```python
from build123d import *

# Parameters (mm, degrees)
SKETCH1_W           = 220
SKETCH1_H           = 220
BOSS_EXTRUDE1_DEPTH = 200
FILLET1_R           = 10
SKETCH2_R           = 30
CUT_EXTRUDE1_DEPTH  = 20
SKETCH3_W           = 80
SKETCH3_H           = 36
CUT_EXTRUDE2_DEPTH  = 20
SKETCH4_W           = 13.191247326
SKETCH4_H           = 23.565374265
CUT_EXTRUDE3_DEPTH  = 10


with BuildPart() as part:
    # Sketch1 → Boss-Extrude1 (new body)
    with BuildSketch(Plane(origin=(0, 0, 0), x_dir=(1, 0, 0), z_dir=(0, 1, 0))):
        Rectangle(SKETCH1_W, SKETCH1_H)
    extrude(amount=BOSS_EXTRUDE1_DEPTH)

    # Fillet1
    fillet1_edges = [part.edges().sort_by_distance(p)[0] for p in [
        (110, 100, 110),
        (-110, 100, 110),
        (-110, 100, -110),
        (110, 100, -110),
    ]]
    fillet(fillet1_edges, radius=FILLET1_R)

    # Sketch2 → Cut-Extrude1 (cut)
    with BuildSketch(Plane.XZ):
        with Locations((0, -50)):
            Circle(SKETCH2_R)
        with Locations((0, 60)):
            Circle(SKETCH2_R)
    extrude(amount=-CUT_EXTRUDE1_DEPTH, mode=Mode.SUBTRACT)

    # Sketch3 → Cut-Extrude2 (cut)
    with BuildSketch(Plane.XY.offset(110)):
        with Locations((0, 162)):
            Rectangle(SKETCH3_W, SKETCH3_H)
    extrude(amount=-CUT_EXTRUDE2_DEPTH, mode=Mode.SUBTRACT)

    # Sketch4 → Cut-Extrude3 (cut)
    with BuildSketch(Plane.ZY.offset(-40)):
        with Locations((100, 164.204493947)):
            Rectangle(SKETCH4_W, SKETCH4_H)
    extrude(amount=-CUT_EXTRUDE3_DEPTH, mode=Mode.SUBTRACT)


solid = part.part
```
Read the model definition and answer for the solid it produces. Units are mm, in the model's axes. A direction names the side the tool comes from. Coordinates: 2 decimals unless noted, no trailing zeros. Write each loop counter-clockwise with the first axis right and the second up, starting at its lowest first coordinate (ties: lowest second). Pieces come first, ordered by that corner, then holes. Notation, with made-up numbers: (88, -3) -> (96, -3) arc R19 ccw to (96, 24) -> close; hole circle Ø8 at (77, -31). An arc over 180 degrees is marked (long way). Answer as a JSON object with one key per item and string values.
Q1. Determine the mould class of faces 1 (the flat face through (-1, 99, -110)), 2 (the flat face through (45, 175.987, 100)), 3 (the flat face through (-40, 162, 100)) for opening direction Z: pulls with the +Z half, pulls with the -Z half, needs draft (parallel to the pull), parting line crosses it, or undercut.
The answers:
{"face 1": "pulls with the -Z half", "face 2": "undercut", "face 3": "needs draft"}
Q2. The part is cut by section A-A on y = 13. Give the vertices of the cut face in (x, z).
The answers:
{"outline": "(-110, -100) arc R10 ccw to (-100, -110) -> (100, -110) arc R10 ccw to (110, -100) -> (110, 100) arc R10 ccw to (100, 110) -> (-100, 110) arc R10 ccw to (-110, 100) -> close; hole circle Ø60 at (0, -50); hole circle Ø60 at (0, 60)"}
Q3. The part is cut by section C-C on x = 0. Give the vertices of the cut face in (y, z).
The answers:
{"outline": "(0, -110) -> (200, -110) -> (200, 110) -> (180, 110) -> (180, 90) -> (144, 90) -> (144, 110) -> (0, 110) -> (0, 90) -> (20, 90) -> (20, 30) -> (0, 30) -> (0, -20) -> (20, -20) -> (20, -80) -> (0, -80) -> close"}
Q4. Consider line 1 (Z direction, x = 0, y = 12.5); line 2 (X direction, y = 18.5, z = 45.5); line 3 (X direction, y = 13, z = 100.5). Determine where each line is inside the solid, lowest interval first. Write a range as [from, to].
The answers:
{"line 1": "z = [-110, -80], [-20, 30], [90, 110]", "line 2": "x = [-110, -26.26], [26.26, 110]", "line 3": "x = [-109.99, 109.99]"}
Q5. A tool of negligible diameter and unlimited length cuts with its end or side. For faces 4 (the flat face through (45, 164, 106.596)), 5 (the flat face through (-1, 180, 100)), 6 (the cylindrical face through (106.99, 101.4, 107.15)), 7 (the flat face through (0, 20, 60)), 8 (the flat face through (-2, 200, -2)), from which of +Z, -Z, +X, -X, +Y, -Y can it reach the whole face along a straight path? Write none if from no direction.
The answers:
{"face 4": "none", "face 5": "+Z", "face 6": "+Z, +X, +Y, -Y", "face 7": "-Y", "face 8": "+Z, -Z, +X, -X, +Y"}
Q6. The part is cut by section D-D on z = -73.5. Give the vertices of the cut face in (x, y).
The answers:
{"outline": "(-110, 0) -> (-18.65, 0) -> (-18.65, 20) -> (18.65, 20) -> (18.65, 0) -> (110, 0) -> (110, 200) -> (-110, 200) -> close"}
Q7. The part is cut by section B-B on z = 60. Give the vertices of the cut face in (x, y), then the cut area to 3 significant figures.
The answers:
{"outline": "(-110, 0) -> (-30, 0) -> (-30, 20) -> (30, 20) -> (30, 0) -> (110, 0) -> (110, 200) -> (-110, 200) -> close", "area": "42,800 mm2"}
